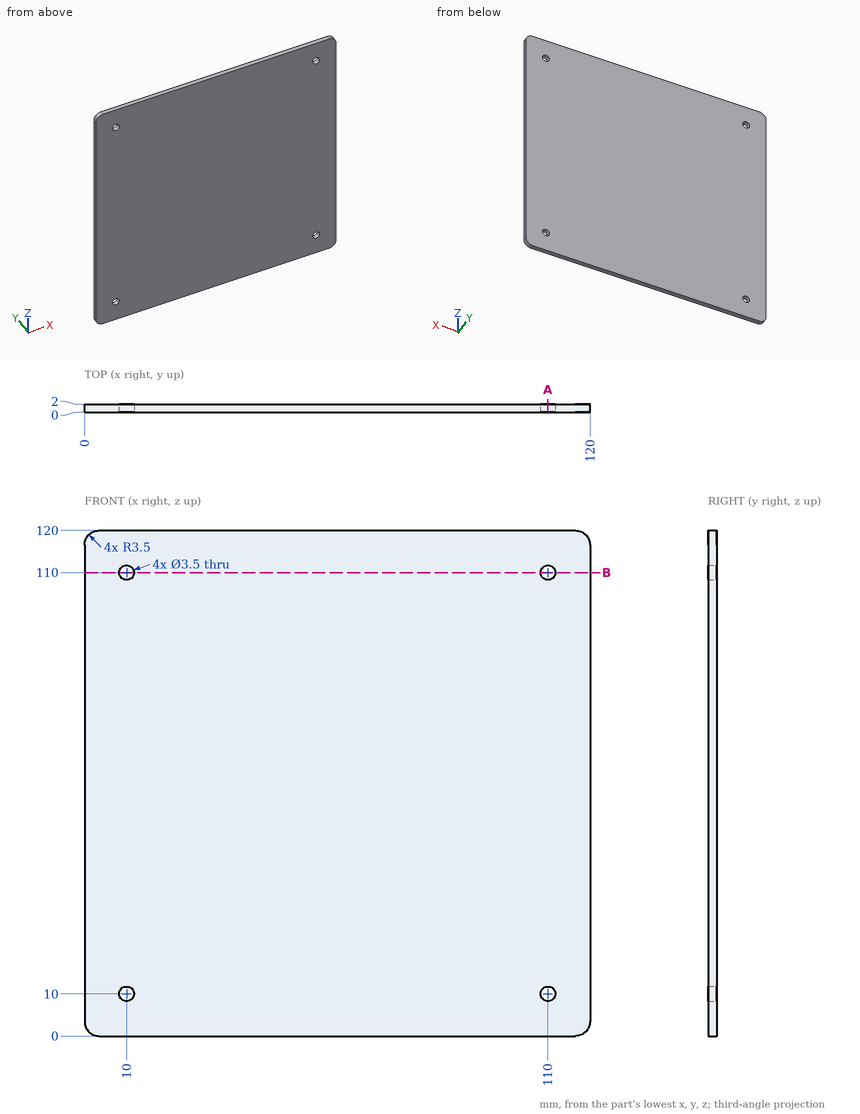
Geometry: see drawing. Coordinates: mm, zero at the bounding-box minimum. Give positions to 0.01 mm unless a question says otherwise; leave off trailing zeros. Order: outer loops, then holes, each group sorted by start corner. A loop starts at its lowest first (then second) coordinate and runs counter-clockwise, first axis right, second up. Notation, with made-up numbers: (-4.75, 46) -> (29.25, 46) arc R13 ccw to (29.25, 60) -> close; hole circle Ø5 at (-32.5, -32). An arc over 180 degrees is marked (long way). Write each question's results on one line, items separated by ' | '. Start each with the question number.
1) Section A-A (x = 110). Return loops of the section in (y, z), then the cut area to 3 significant figures.
2) Section B-B (z = 110). Return loops of the section in (x, y), then the cut area to 3 significant figures.
3) Line query: line 1 (X direction, y = 0.9, z = 10). Output: solid intervals per line, ascending. Write a range as from..to.
4) First-contact query: pin 1 (3 mm diameter, centred on x = 10, z = 10, fed in from +Y). Flat tip, straight axial feed; report the tip coordinate or a pass-through.
Calculated:
1) outline: (0, 0) -> (2, 0) -> (2, 8.25) -> (0, 8.25) -> close; (0, 11.75) -> (2, 11.75) -> (2, 108.25) -> (0, 108.25) -> close; (0, 111.75) -> (2, 111.75) -> (2, 120) -> (0, 120) -> close | area: 226 mm2
2) outline: (0, 0) -> (8.25, 0) -> (8.25, 2) -> (0, 2) -> close; (11.75, 0) -> (108.25, 0) -> (108.25, 2) -> (11.75, 2) -> close; (111.75, 0) -> (120, 0) -> (120, 2) -> (111.75, 2) -> close | area: 226 mm2
3) line 1: 0..8.25, 11.75..108.25, 111.75..120
4) pin 1: through
